```python
from build123d import *

# Parameters (mm, degrees)
EXTRUDE_1_DEPTH = 1
SKETCH_9_W      = 0.82
SKETCH_9_H      = 10.5
EXTRUDE_4_DEPTH = 10.5


with BuildPart() as part:
    # Sketch 1 → Extrude 1 (new body)
    with BuildSketch(Plane.XY):
        with BuildLine():
            Line((17.75, -8.875), (6.75, -8.875))
            ThreePointArc((6.75, -8.875), (5.335786438, -8.289213562), (4.75, -6.875))
            Line((4.75, -6.875), (4.75, 14.125))
            ThreePointArc((4.75, 14.125), (5.335786438, 15.539213562), (6.75, 16.125))
            Line((6.75, 16.125), (17.75, 16.125))
            ThreePointArc((17.75, 16.125), (19.164213562, 15.539213562), (19.75, 14.125))
            Line((19.75, 14.125), (19.75, -6.875))
            ThreePointArc((19.75, -6.875), (19.164213562, -8.289213562), (17.75, -8.875))
        make_face()
    extrude(amount=EXTRUDE_1_DEPTH)



with BuildPart() as body_2:
    # Sketch 9 → Revolve 2 (revolve)
    with BuildSketch(Plane.XY.offset(1.5), mode=Mode.PRIVATE) as revolve_2_sk:
        with Locations((4.34, 8.875)):
            Rectangle(SKETCH_9_W, SKETCH_9_H)
    revolve(revolve_2_sk.sketch.rotate(Axis((3.25, 14.125, 1.5), (0, -1, 0)), 180), axis=Axis((3.25, 14.125, 1.5), (0, -1, 0)))


with BuildPart() as part_1:
    add(part.part)

    add(body_2.part)  # Extrude 4 merges body 2
    # Sketch 11 → Extrude 4 (add)
    with BuildSketch(Plane(origin=(0, 14.125, 0), x_dir=(1, 0, 0), z_dir=(0, 1, 0))):
        with BuildLine():
            Line((4.75, -1), (4.75, -0.82))
            Line((4.75, -0.82), (4.587011593, -0.82))
            ThreePointArc((4.587011593, -0.82), (4.628553577, -0.908738606), (4.664213562, -1))
            Line((4.664213562, -1), (4.75, -1))
        make_face()
        with BuildLine():
            Line((4.75, -0.82), (4.75, 0))
            Line((4.75, 0), (3.25, 0))
            ThreePointArc((3.25, 0), (4.034219357, -0.221328815), (4.587011593, -0.82))
            Line((4.587011593, -0.82), (4.75, -0.82))
        make_face()
    extrude(amount=-EXTRUDE_4_DEPTH)


solid = part_1.part
```
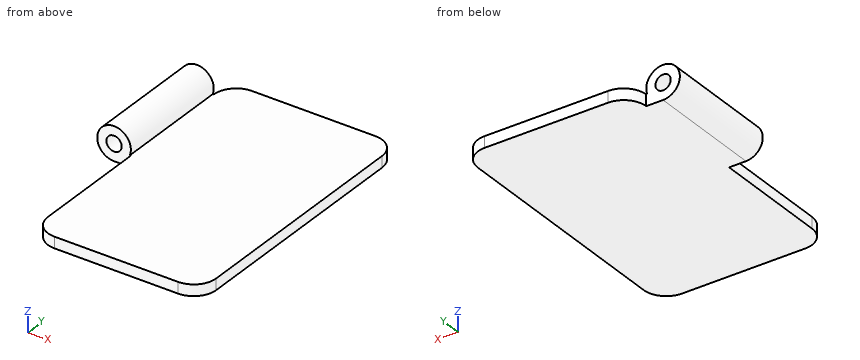
CAD build for the part. Positions are in the model's coordinates, mm. Round coordinates to 2 decimals unless told otherwise and drop trailing zeros. Write each loop counter-clockwise with the first axis right and the second up, starting at its lowest first coordinate (ties: lowest second). Pieces come first, ordered by that corner, then holes. Notation, with made-up numbers: (37.25, 4.25) - (84.25, 4.25) arc R19 cw to (84.25, 14.25) - close; hole circle Ø5 at (35.5, -11.5). An arc over 180 degrees is marked (long way). Write item = value, one per line. Start each with the question number.
Q1. Band-saw the part on D-D (y = 1). Give the cut face in (x, z), then the cut area to 3 significant figures.
Q2. Probe L1, parallel to Z at x = 3.25, y = 7.75; L2, parallel to X at y = 11.25, z = 1.5; L3, parallel to Z at x = 11.5, y = -5.75. List the from-to ranges inside material, lowest first. Write a range as from..to.
Q3. Drop flat-ended pins along their axis: pin 1 (1.5 mm diameter, centred on x = 3.5, z = 1.5, fed in from -Y) (3 decimals); pin 2 (4 mm diameter, centred on x = 6, y = 11, fed in from +Z); pin 3 (8 mm diameter, centred on x = 10.5, y = 0, fed in from +Z); pin 4 (1.5 mm diameter, centred on x = 12.5, z = 2.5, fed in from +Y). Give the stop position or say it passes through.
Q4. Band-saw the part on A-A (z = 1.5). Give the cut face in (x, y) (3 decimals).
Q5. Band-saw the part on B-B (y = 11.25). Give the cut face in (x, z), then the cut area to 3 significant figures.
Q6. Band-saw the part on C-C (x = 8.25). Give the cut face in (y, z) (3 decimals).
Answers below:
q1.outline = (4.75, 0) - (19.75, 0) - (19.75, 1) - (4.75, 1) - close
q1.area = 15.0 mm2
q2.L1 = 0..0.82, 2.18..3
q2.L2 = 1.75..2.57, 3.93..4.75
q2.L3 = 0..1
q3.pin_1 = 3.625
q3.pin_2 = 2.8
q3.pin_3 = 1
q3.pin_4 = through
q4.outline = (1.75, 3.625) - (2.57, 3.625) - (2.57, 14.125) - (1.75, 14.125) - close; (3.93, 3.625) - (4.75, 3.625) - (4.75, 14.125) - (3.93, 14.125) - close
q5.outline = (3.25, 0) - (19.75, 0) - (19.75, 1) - (4.66, 1) arc R1.5 ccw (long way) to start; hole circle Ø1.36 at (3.25, 1.5)
q5.area = 21.1 mm2
q6.outline = (-8.875, 0) - (16.125, 0) - (16.125, 1) - (-8.875, 1) - close
